```python
from build123d import *

# Parameters (mm, degrees)
SKETCH_1_W               = 15
SKETCH_1_H               = 17.8
SKETCH_1_R               = 3
SKETCH_1_W_2             = 6
SKETCH_1_H_2             = 2.9
SKETCH_1_R_2             = 1.7
EXTRUDE_1_DEPTH          = 3.2
SKETCH_1_3_W             = 15
SKETCH_1_3_H             = 17.8
SKETCH_1_3_R             = 3
SKETCH_1_3_W_2           = 6
SKETCH_1_3_H_2           = 2.9
EXTRUDE_2_DEPTH          = 2.2
EXTRUDE_START            = -2.2
SKETCH_1_4_W             = 15
SKETCH_1_4_H             = 17.8
SKETCH_1_4_R             = 3
SKETCH_1_4_W_2           = 6
SKETCH_1_4_H_2           = 2.9
EXTRUDE_3_DEPTH          = 7.7
CUT_EXTRUDE_1_DEPTH      = 16.279725128
CUT_EXTRUDE_1_DEPTH_BACK = 16.279725128
SKETCH_2_R               = 1.7
FILLET_1_R               = 2


with BuildPart() as part:
    # 草图1 → 凸台-拉伸1 (new body)
    # profile 1 of 4: a face of its own
    with BuildSketch(Plane.XY):
        Rectangle(SKETCH_1_W, SKETCH_1_H)
        Circle(SKETCH_1_R, mode=Mode.SUBTRACT)
        with Locations((0, -5.45)):
            Rectangle(SKETCH_1_W_2, SKETCH_1_H_2, mode=Mode.SUBTRACT)
        with Locations((0, 5.45)):
            Rectangle(SKETCH_1_W_2, SKETCH_1_H_2, mode=Mode.SUBTRACT)
    # profile 2 of 4: a face of its own
    with BuildSketch(Plane.XY):
        Circle(SKETCH_1_R)
        Circle(SKETCH_1_R_2, mode=Mode.SUBTRACT)
    # profile 3 of 4: a face of its own
    with BuildSketch(Plane.XY):
        with Locations((0, 5.45)):
            Rectangle(SKETCH_1_W_2, SKETCH_1_H_2)
    # profile 4 of 4: a face of its own
    with BuildSketch(Plane.XY):
        with Locations((0, -5.45)):
            Rectangle(SKETCH_1_W_2, SKETCH_1_H_2)
    extrude(amount=EXTRUDE_1_DEPTH)

    # 草图1<3> → 凸台-拉伸2 (add)
    # profile 1 of 3: a face of its own
    with BuildSketch(Plane.XY):
        Rectangle(SKETCH_1_3_W, SKETCH_1_3_H)
        Circle(SKETCH_1_3_R, mode=Mode.SUBTRACT)
        with Locations((0, -5.45)):
            Rectangle(SKETCH_1_3_W_2, SKETCH_1_3_H_2, mode=Mode.SUBTRACT)
        with Locations((0, 5.45)):
            Rectangle(SKETCH_1_3_W_2, SKETCH_1_3_H_2, mode=Mode.SUBTRACT)
    # profile 2 of 3: a face of its own
    with BuildSketch(Plane.XY):
        with Locations((0, 5.45)):
            Rectangle(SKETCH_1_3_W_2, SKETCH_1_3_H_2)
    # profile 3 of 3: a face of its own
    with BuildSketch(Plane.XY):
        with Locations((0, -5.45)):
            Rectangle(SKETCH_1_3_W_2, SKETCH_1_3_H_2)
    extrude(amount=-EXTRUDE_2_DEPTH)

    # 草图1<4> → 凸台-拉伸3 (add)
    with BuildSketch(Plane.XY.offset(EXTRUDE_START)):
        Rectangle(SKETCH_1_4_W, SKETCH_1_4_H)
        Circle(SKETCH_1_4_R, mode=Mode.SUBTRACT)
        with Locations((0, -5.45)):
            Rectangle(SKETCH_1_4_W_2, SKETCH_1_4_H_2, mode=Mode.SUBTRACT)
        with Locations((0, 5.45)):
            Rectangle(SKETCH_1_4_W_2, SKETCH_1_4_H_2, mode=Mode.SUBTRACT)
    extrude(amount=-EXTRUDE_3_DEPTH)

    # 草图2 → 切除-拉伸1 (cut, two sides: drawn at the far end of the back side and taken through both)
    with BuildSketch(Plane(origin=(0, 0, 0), x_dir=(1, 0, 0), z_dir=(0, 1, 0)).offset(-CUT_EXTRUDE_1_DEPTH_BACK)):
        with Locations(Location((0, 6.2, 0), (0, 0, 270))):
            Circle(SKETCH_2_R)
    extrude(amount=CUT_EXTRUDE_1_DEPTH + CUT_EXTRUDE_1_DEPTH_BACK, mode=Mode.SUBTRACT)

    # 圆角1
    fillet_1_edges = [part.edges().sort_by_distance(p)[0] for p in [
        (-7.5, -8.9, -3.35),
        (-7.5, 8.9, -3.35),
        (7.5, 8.9, -3.35),
        (7.5, -8.9, -3.35),
        (-7.5, 0, -9.9),
        (7.5, 0, -9.9),
    ]]
    fillet(fillet_1_edges, radius=FILLET_1_R)


solid = part.part
```
Work out the finished part from the listing and answer in its coordinate system (mm). A direction names the side the tool comes from. Coordinates: 2 decimals unless noted, no trailing zeros. Write each loop counter-clockwise with the first axis right and the second up, starting at its lowest first coordinate (ties: lowest second). Pieces come first, ordered by that corner, then holes.
Q1. Which of the six approach directions +Z, -Z, +X, -X, +Y, -Y give full straight-line access (tool end or side, diameter ignored) to faces 1 (the face through (0, -5, -2.2)), 2 (the face through (-0.65, -7.91, -4.63))?
Q2. A cutting plane is placed at C-C, the plane z = -2.5. Give the vertices of the cut face in (x, y), then the cut area to 3 significant figures.
Q3. Find the intervals of material crossed by line 1 (Z direction, x = 0, y = 7.75); line 2 (Y direction, x = 1.5, z = -7.5); line 3 (X direction, y = -4.25, z = -3.25), in increasing order.
Q4. Each of these flat-tipped pins is pushed along its axis until it touches: pin 1 Ø5 at (x, y) = (0, 0) entering from -Z; pin 2 Ø2 at (x, z) = (0, -6.2) entering from -Y; pin 3 Ø0.9 at (x, y) = (1, -5) entering from -Z. Where does it stop, or does it pass through?
Q5. A cutting plane is placed at D-D, the plane z = 2.5. Give the vertices of the cut face in (x, y).
Q6. A cutting plane is placed at B-B, the plane y = 6.25. Give the vertices of the cut face in (x, z).
Q7. Determine the mould class of faces 3 (the face through (7.5, 0, -2)), 4 (the face through (-3, -2, -9.9)), 5 (the face through (0, -4, -4)), 6 (the face through (3, 5, -6)) for opening direction X: released by +X, released by -X, zero draft, split by the parting line, or undercut.
Findings below:
1. face 1: -Z
1. face 2: +Y, -Y
2. outline: (-7.5, -6.9) arc R2 ccw to (-5.5, -8.9) - (5.5, -8.9) arc R2 ccw to (7.5, -6.9) - (7.5, 6.9) arc R2 ccw to (5.5, 8.9) - (-5.5, 8.9) arc R2 ccw to (-7.5, 6.9) - close; hole (-3, -6.9) - (3, -6.9) - (3, -4) - (-3, -4) - close; hole circle Ø6 at (0, 0); hole (-3, 4) - (3, 4) - (3, 6.9) - (-3, 6.9) - close
2. area: 200 mm2
3. line 1: z = -9.9 to -7.9, -4.5 to 3.2
3. line 2: y = -8.9 to -6.9, -4 to -2.6, 2.6 to 4, 6.9 to 8.9
3. line 3: x = -7.5 to -3, 3 to 7.5
4. pin 1: stops at z = 0
4. pin 2: passes through
4. pin 3: stops at z = -2.2
5. outline: (-7.5, -6.9) arc R2 ccw to (-5.5, -8.9) - (5.5, -8.9) arc R2 ccw to (7.5, -6.9) - (7.5, 6.9) arc R2 ccw to (5.5, 8.9) - (-5.5, 8.9) arc R2 ccw to (-7.5, 6.9) - close; hole circle Ø3.4 at (0, 0)
6. outline: (-7.5, -7.9) arc R2 ccw to (-5.5, -9.9) - (-3, -9.9) - (-3, -2.2) - (3, -2.2) - (3, -9.9) - (5.5, -9.9) arc R2 ccw to (7.5, -7.9) - (7.5, 3.2) - (-7.5, 3.2) - close
7. face 3: released by +X
7. face 4: zero draft
7. face 5: undercut
7. face 6: undercut
